Read the model definition and answer for the solid it produces. Units are mm, in the model's axes. A direction names the side the tool comes from. Coordinates: 2 decimals unless noted, no trailing zeros. Write each loop counter-clockwise with the first axis right and the second up, starting at its lowest first coordinate (ties: lowest second). Pieces come first, ordered by that corner, then holes.
(1) The part is cut by section B-B, the plane x = 20. Determine the outline of the cut face in (y, z).
(2) Determine the mould class of faces 1 (the flat face through (-35.63, -21.55, 19.52)), 2 (the flat face through (37.626, -21.548, 6.274)), 3 (the flat face through (2, -42.5, 13)) for opening direction X: pulls with the +X half, pulls with the -X half, needs draft (parallel to the pull), parting line crosses it, or undercut.
(3) The part is cut by section D-D, the plane x = -27.5. Determine the outline of the cut face in (y, z), and give its area (3 significant figures).
(4) Which of the six approach directions +Z, -Z, +X, -X, +Y, -Y give full straight-line access (tool end or side, diameter ignored) to faces 4 (the flat face through (29.936, -21.548, -0.866)), 5 (the flat face through (2, 0, 13))?
(5) The part is cut by section A-A, the plane y = -40. Determine the outline of the cut face in (x, z).
(6) Given pin 1 (3 mm diameter, centred on x = -3, y = -12, fed in from -Z); pin 2 (1.5 mm diameter, centred on y = -24, z = 4, fed in from -X); pin 3 (5 mm diameter, centred on y = -15, z = 20.5, fed in from -X), each flat-ended and moving along its own axis, determine where each tip first touches the part or whether it passes through.
(7) The part is cut by section C-C, the plane z = 17.5. Determine the outline of the cut face in (x, y), and give its area (3 significant figures).
(8) Straight lines are drawn through the part: line 1 along Z through (x, y) = (16, -13); line 2 along Z through (x, y) = (-31, -25.5); line 3 along Z through (x, y) = (-22.5, -34). For each, find the intervals that lie inside material, in ascending order.
```python
from build123d import *

# Parameters (mm, degrees)
F0_W     = 180
F0_H     = 80
F1_DEPTH = 85
F3_DEPTH = 85.001
F5_DEPTH = 85.001
F6_SCALE = 0.5


with BuildPart() as f1:
    # F0 (on Front) → F1 (new body)
    with BuildSketch(Plane.XZ):
        with Locations((4.7223418951, 11.9884983084)):
            Rectangle(F0_W, F0_H)
    extrude(amount=F1_DEPTH)

    # F2 (on face) → F3 (cut, through all)
    with BuildSketch(Plane.XZ.offset(85)):
        Polygon((-46.0070036352, -28.0115016916), (-85.2776581049, 51.9884983084), (-85.2776581049, -28.0115016916), align=None)
        Polygon((94.7223418951, -28.0115016916), (94.7223418951, 51.9884983084), (55.2294403315, -28.0115016916), align=None)
    extrude(amount=-F3_DEPTH, mode=Mode.SUBTRACT)

    # F4 (on face) → F5 (cut, through all)
    with BuildSketch(Plane.XZ.offset(85)):
        Polygon((-74.7092828557, 46.072713804), (-67.7043439121, 31.8026405634), (76.6995772719, 31.8026405634), (83.6467270564, 46.072713804), align=None)
        Polygon((73.4329734772, 25.2924152588), (-64.5085838063, 25.2924152588), (-38.3425875008, -28.0115016916), (46.6869287193, -28.0115016916), align=None)
    extrude(amount=-F5_DEPTH, mode=Mode.SUBTRACT)


with BuildPart() as f1_1:
    # F6: moved
    add(f1.part.scale(F6_SCALE))


solid = f1_1.part
```
Computed:
1. outline: (-42.5, 12.65) - (0, 12.65) - (0, 15.9) - (-42.5, 15.9) - close; (-42.5, 23.04) - (0, 23.04) - (0, 25.99) - (-42.5, 25.99) - close
2. face 1: undercut
2. face 2: pulls with the +X half
2. face 3: needs draft
3. outline: (-42.5, -4.85) - (0, -4.85) - (0, 2.96) - (-42.5, 2.96) - close; (-42.5, 12.65) - (0, 12.65) - (0, 15.9) - (-42.5, 15.9) - close; (-42.5, 23.04) - (0, 23.04) - (0, 25.99) - (-42.5, 25.99) - close
3. area: 596 mm2
4. face 4: +Y, -Y
4. face 5: +Z, -Z, +X, -X, +Y
5. outline: (-42.64, 25.99) - (-23, -14.01) - (-19.17, -14.01) - (-32.25, 12.65) - (36.72, 12.65) - (23.34, -14.01) - (27.61, -14.01) - (47.36, 25.99) - close; hole (-37.35, 23.04) - (-33.85, 15.9) - (38.35, 15.9) - (41.82, 23.04) - close
6. pin 1: stops at z = 12.65
6. pin 2: stops at x = -32.21
6. pin 3: stops at x = -41.17
7. outline: (-38.47, -42.5) - (-34.64, -42.5) - (-34.64, 0) - (-38.47, 0) - close; (39.13, -42.5) - (43.17, -42.5) - (43.17, 0) - (39.13, 0) - close
7. area: 335 mm2
8. line 1: z = 12.65 to 15.9, 23.04 to 25.99
8. line 2: z = 2.28 to 10.09, 12.65 to 15.9, 23.04 to 25.99
8. line 3: z = -14.01 to -7.22, 12.65 to 15.9, 23.04 to 25.99
